Input: part model. Units: mm. Frame: model coordinates. Face numbers are marked on the shaded views. Coordinates: 2 decimals unless noted, no trailing zeros. Loops run counter-clockwise (first coordinate to the right, second up) from the corner with the lowest first, then second, coordinate; pieces in that order, holes last.
(1) Contact query for a flat-ended pin moving along its axis: P1, Ø12, axis at x = -38.1, y = 0, coming from the +Z side. Output: stop coordinate, or through.
(2) Mould query, pull axis Y, two halves, no side actions, for the marked faces 1, 2, 3 and 4. Classes: released by +Y, released by -Y, zero draft, split by the parting line, or undercut.
(3) Section D-D, the plane y = 0. Return loops of the section in (x, z).
(4) Section A-A, the plane x = 13. Return loops of the section in (y, z).
(5) Section C-C, the plane z = 5. Give the number of separate pieces and of enclosed holes in the cut face, then the cut area to 3 significant figures.
(6) Section B-B, the plane y = -13. Return loops of the section in (x, z), then the cut area to 3 significant figures.
(7) Line query: L1, parallel to Y at x = -13, z = 2.25; L2, parallel to X at y = -13, z = 4.25; L3, parallel to Y at x = 0, z = 3.5. Output: solid intervals per line, ascending.
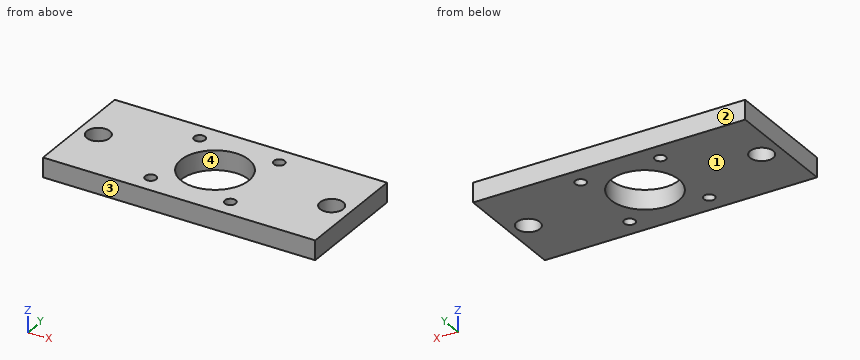
```python
from build123d import *

# Parameters (mm, degrees)
F1_DEPTH = 6.35
F2_D     = 3.6
F3_D     = 7.5438
F4_D     = 22.225


# Not quite as in the source:
# - a length typed as a fraction of an inch, garbled in the dataset ("3 / 203.2 mm" for 3/8 in), is restored


with BuildPart() as f1:
    # F0 (on Top) → F1 (new body)
    with BuildSketch(Plane.XY):
        Polygon((44.45, 13), (44.45, 19.05), (-44.45, 19.05), (-44.45, -19.05), (44.45, -19.05), align=None)
    extrude(amount=F1_DEPTH)

    # F2 (through all)
    with Locations(Plane(origin=(0, 0, 0), x_dir=(1, 0, 0), z_dir=(0, 0, -1))):
        with Locations((-13, -13), (13, -13), (13, 13), (-13, 13)):
            Hole(F2_D / 2)

    # F3 (through all)
    with Locations(Plane(origin=(0, 0, 0), x_dir=(1, 0, 0), z_dir=(0, 0, -1))):
        with Locations((-38.1, 0), (38.1, 0)):
            Hole(F3_D / 2)

    # F4 (through all)
    with Locations(Plane(origin=(0, 0, 0), x_dir=(1, 0, 0), z_dir=(0, 0, -1))):
        with Locations((0, 0)):
            Hole(F4_D / 2)


solid = f1.part
```
Report:
1. P1: stops at z = 6.35
2. face 1: zero draft
2. face 2: released by +Y
2. face 3: released by -Y
2. face 4: undercut
3. outline: (-44.45, 0) - (-41.87, 0) - (-41.87, 6.35) - (-44.45, 6.35) - close; (-34.33, 0) - (-11.11, 0) - (-11.11, 6.35) - (-34.33, 6.35) - close; (11.11, 0) - (34.33, 0) - (34.33, 6.35) - (11.11, 6.35) - close; (41.87, 0) - (44.45, 0) - (44.45, 6.35) - (41.87, 6.35) - close
4. outline: (-19.05, 0) - (-14.8, 0) - (-14.8, 6.35) - (-19.05, 6.35) - close; (-11.2, 0) - (11.2, 0) - (11.2, 6.35) - (-11.2, 6.35) - close; (14.8, 0) - (19.05, 0) - (19.05, 6.35) - (14.8, 6.35) - close
5. separate pieces: 1
5. enclosed holes: 7
5. area: 2,870 mm2
6. outline: (-44.45, 0) - (-14.8, 0) - (-14.8, 6.35) - (-44.45, 6.35) - close; (-11.2, 0) - (11.2, 0) - (11.2, 6.35) - (-11.2, 6.35) - close; (14.8, 0) - (44.45, 0) - (44.45, 6.35) - (14.8, 6.35) - close
6. area: 519 mm2
7. L1: y = -19.05 to -14.8, -11.2 to 11.2, 14.8 to 19.05
7. L2: x = -44.45 to -14.8, -11.2 to 11.2, 14.8 to 44.45
7. L3: y = -19.05 to -11.11, 11.11 to 19.05
